```python
from build123d import *

# Parameters (mm, degrees)
BOSS_EXTRUDE1_DEPTH             = 227.5
TAP_DRILL_FOR_M5X0_8_TAP1_D     = 5
TAP_DRILL_FOR_M5X0_8_TAP1_DEPTH = 10
TAP_DRILL_FOR_M5X0_8_TAP2_D     = 5
TAP_DRILL_FOR_M5X0_8_TAP2_DEPTH = 10
TAP_DRILL_FOR_M5X0_8_TAP3_D     = 5
TAP_DRILL_FOR_M5X0_8_TAP3_DEPTH = 10
TAP_DRILL_FOR_M5X0_8_TAP4_D     = 5
TAP_DRILL_FOR_M5X0_8_TAP4_DEPTH = 10
TAP_DRILL_FOR_M5X0_8_TAP5_D     = 5
TAP_DRILL_FOR_M5X0_8_TAP5_DEPTH = 5.5
TAP_DRILL_FOR_M5X0_8_TAP6_D     = 5
TAP_DRILL_FOR_M5X0_8_TAP6_DEPTH = 5.5
SKETCH18_R                      = 1.5
CUT_EXTRUDE2_DEPTH              = 29


with BuildPart() as part:
    # Sketch1 → Boss-Extrude1 (new body)
    with BuildSketch(Plane.XY):
        Polygon((44.5, 5.5), (-44.5, 5.5), (-44.5, 14.835), (-50.17, 14.835), (-50.17, 20.5), (-59.5, 20.5), (-59.5, 0), (59.5, 0), (59.5, 20.5), (50.17, 20.5), (50.17, 14.835), (44.5, 14.835), align=None)
    extrude(amount=BOSS_EXTRUDE1_DEPTH)

    # Tap Drill for M5x0.8 Tap1
    with Locations(Plane.XY.offset(227.5)):
        with Locations((52, 8), (-52, 8)):
            Hole(TAP_DRILL_FOR_M5X0_8_TAP1_D / 2, depth=TAP_DRILL_FOR_M5X0_8_TAP1_DEPTH)

    # Tap Drill for M5x0.8 Tap2
    with Locations(Plane(origin=(0, 0, 0), x_dir=(-1, 0, 0), z_dir=(0, 0, -1))):
        with Locations((52, 8), (-52, 8)):
            Hole(TAP_DRILL_FOR_M5X0_8_TAP2_D / 2, depth=TAP_DRILL_FOR_M5X0_8_TAP2_DEPTH)

    # Tap Drill for M5x0.8 Tap3
    with Locations(Plane(origin=(59.5, 0, 0), x_dir=(0, 0, -1), z_dir=(1, 0, 0))):
        with Locations((-193.75, 10), (-153.75, 10), (-113.75, 10), (-73.75, 10), (-33.75, 10)):
            Hole(TAP_DRILL_FOR_M5X0_8_TAP3_D / 2, depth=TAP_DRILL_FOR_M5X0_8_TAP3_DEPTH)

    # Tap Drill for M5x0.8 Tap4
    with Locations(Plane.ZY.offset(59.5)):
        with Locations((193.75, 10), (153.75, 10), (113.75, 10), (73.75, 10), (33.75, 10)):
            Hole(TAP_DRILL_FOR_M5X0_8_TAP4_D / 2, depth=TAP_DRILL_FOR_M5X0_8_TAP4_DEPTH)

    # Tap Drill for M5x0.8 Tap5
    with Locations(Plane(origin=(59.5, 0, 0), x_dir=(0, 0, -1), z_dir=(1, 0, 0))):
        with Locations((-177.5, 12.346163158), (-132.5, 12.346163158), (-95, 12.346163158), (-50, 12.346163158)):
            Hole(TAP_DRILL_FOR_M5X0_8_TAP5_D / 2, depth=TAP_DRILL_FOR_M5X0_8_TAP5_DEPTH)

    # Tap Drill for M5x0.8 Tap6
    with Locations(Plane.ZY.offset(59.5)):
        with Locations((50, 12.346163158), (95, 12.346163158), (132.5, 12.346163158), (177.5, 12.346163158)):
            Hole(TAP_DRILL_FOR_M5X0_8_TAP6_D / 2, depth=TAP_DRILL_FOR_M5X0_8_TAP6_DEPTH)

    # Sketch18 → Cut-Extrude2 (cut)
    with BuildSketch(Plane(origin=(59.5, 0, 0), x_dir=(0, 0, -1), z_dir=(1, 0, 0))):
        with Locations(Location((-193.75, 17.6675, 0), (0, 0, 90))):
            Circle(SKETCH18_R)
        with Locations(Location((-153.75, 17.6675, 0), (0, 0, 90))):
            Circle(SKETCH18_R)
        with Locations(Location((-113.75, 17.6675, 0), (0, 0, 90))):
            Circle(SKETCH18_R)
        with Locations(Location((-73.75, 17.6675, 0), (0, 0, 90))):
            Circle(SKETCH18_R)
        with Locations(Location((-33.704207464, 17.6675, 0), (0, 0, 90))):
            Circle(SKETCH18_R)
    extrude(amount=-CUT_EXTRUDE2_DEPTH, mode=Mode.SUBTRACT)


solid = part.part
```
Could you check a few things on this model? Use its own coordinates, in mm. A direction names the side the tool comes from. Round coordinates to 2 decimals unless told otherwise and drop trailing zeros. Loops run counter-clockwise (first coordinate to the right, second up) from the corner with the lowest first, then second, coordinate; pieces in that order, holes last.
Q1. On a 3-axis mill with a long thin cutter (end or side, diameter ignored), from which of +Z, -Z, +X, -X, +Y, -Y can I reach the whole of each face in a straight line? I mean faces 5 (the cylindrical face through (54.43, 9.04, 196.06)), 6 (the flat face through (-49.5, 10, 74)), 7 (the flat face through (-47, 14.835, 112)). Say none if no direction works.
Q2. I want a section at B-B (x = -37.5). Write out the boundary of the cut face in (y, z).
Q3. I want a section at A-A (z = 101.5). Write out the boundary of the cut face in (x, y) (3 decimals).
Q4. For P1, Ø1.5, axis at y = 12.5, z = 133, coming from the +X side; P2, Ø3, axis at y = 10, z = 73.75, coming from the -X side; P3, Ø6, axis at x = 21.5, z = 98.5, coming from the +Y side, each with a flat end and sliding along its axis, tell me the tip position at first contact or that it passes through.
Q5. I want a section at C-C (z = 177.5). Write out the boundary of the cut face in (x, y) (3 decimals), and give its area (3 significant figures).
Q6. Thinking about a two-plate mould opening in Z: for faces 1 (the cylindrical face through (54.31, 7.04, 5.07)), 2 (the cylindrical face through (56.712, 13.097, 52.385)), 3 (the flat face through (0, 5, 0)), 4 (the flat face through (0, 5, 227.5)), which applies, pulls with the +Z half, pulls with the -Z half, needs draft (parallel to the pull), parting line crosses it, or undercut?
Q7. Please list where these lines run through material, in increasing order: L1, parallel to X at y = 18.25, z = 38.5; L2, parallel to X at y = 14.5, z = 78.5; L3, parallel to Y at x = -57, z = 177.
Answer below:
1. face 5: +X
1. face 6: -X
1. face 7: +Z, -Z, +Y
2. outline: (0, 0) - (5.5, 0) - (5.5, 227.5) - (0, 227.5) - close
3. outline: (-59.5, 0) - (59.5, 0) - (59.5, 20.5) - (50.17, 20.5) - (50.17, 14.835) - (44.5, 14.835) - (44.5, 5.5) - (-44.5, 5.5) - (-44.5, 14.835) - (-50.17, 14.835) - (-50.17, 20.5) - (-59.5, 20.5) - close
4. P1: stops at x = 54
4. P2: stops at x = -49.5
4. P3: stops at y = 5.5
5. outline: (-59.5, 0) - (59.5, 0) - (59.5, 9.846) - (54, 9.846) - (54, 14.846) - (59.5, 14.846) - (59.5, 20.5) - (50.17, 20.5) - (50.17, 14.835) - (44.5, 14.835) - (44.5, 5.5) - (-44.5, 5.5) - (-44.5, 14.835) - (-50.17, 14.835) - (-50.17, 20.5) - (-59.5, 20.5) - (-59.5, 14.846) - (-54, 14.846) - (-54, 9.846) - (-59.5, 9.846) - close
5. area: 985 mm2
6. face 1: needs draft
6. face 2: undercut
6. face 3: pulls with the -Z half
6. face 4: pulls with the +Z half
7. L1: x = -59.5 to -50.17, 50.17 to 59.5
7. L2: x = -59.5 to -44.5, 44.5 to 59.5
7. L3: y = 0 to 9.9, 14.8 to 20.5
